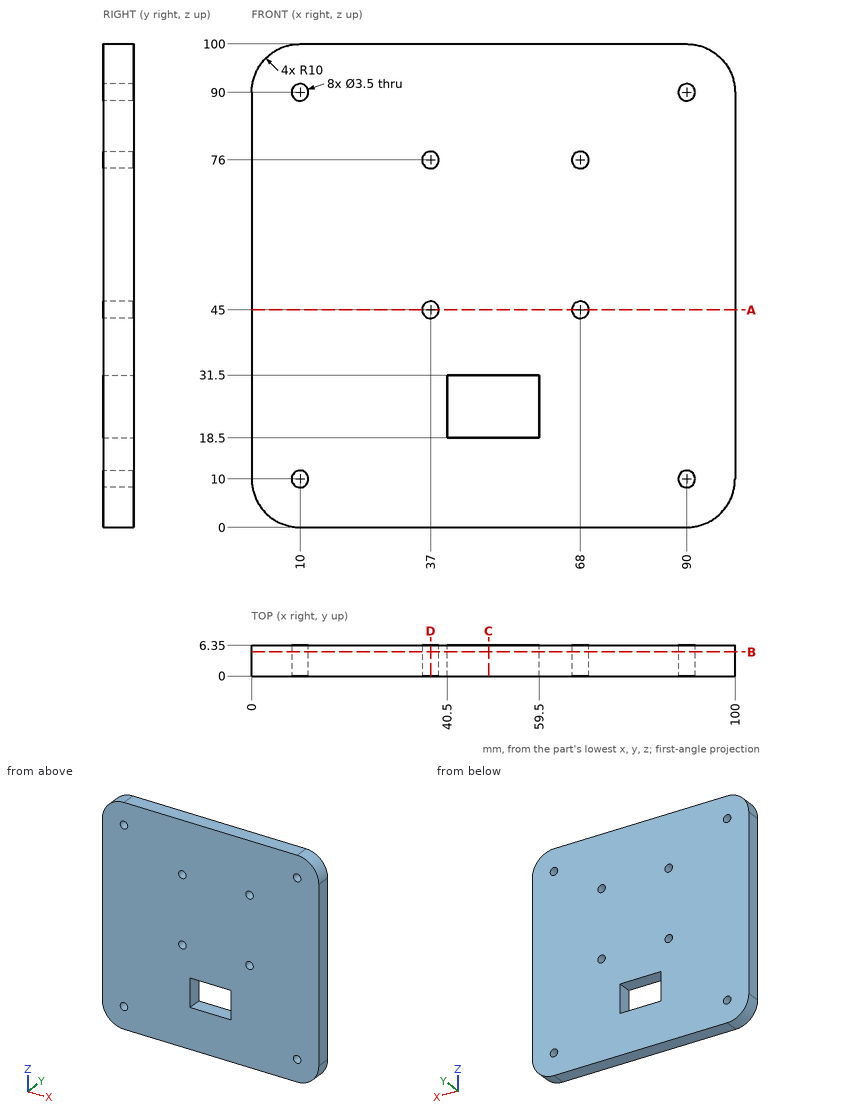
Here's the drawing with two shaded views (mm, measured from the low corner). I have some questions. Coordinates: 2 decimals unless noted, no trailing zeros. Order: outer loops, then holes, each group sorted by start corner. A loop starts at its lowest first (then second) coordinate and runs counter-clockwise, first axis right, second up.
Q1. Suppose I cut it at A-A on z = 45. Please give me the cut outline in (x, y).
Q2. Will these pins go through, and if not, where does the flat tip stop? pin 1 (3 mm diameter, centred on x = 37, z = 45, fed in from -Y); pin 2 (4 mm diameter, centred on x = 68, z = 45, fed in from +Y).
Q3. Please list where these lines run through material, in increasing order: L1, parallel to X at y = 4.25, z = 76; L2, parallel to Z at x = 68, y = 3.75; L3, parallel to X at y = 2.5, z = 27.5.
Q4. Suppose I cut it at C-C on x = 49. Please give me the cut outline in (y, z), and give its area (3 significant figures).
Q5. Suppose I cut it at D-D on x = 37. Please give me the cut outline in (y, z).
Q6. Suppose I cut it at B-B on y = 5. Give the number of separate pieces and of enclosed holes in the cut face, and give its area (3 significant figures).
Answer:
1. outline: (0, 0) - (35.25, 0) - (35.25, 6.35) - (0, 6.35) - close; (38.75, 0) - (66.25, 0) - (66.25, 6.35) - (38.75, 6.35) - close; (69.75, 0) - (100, 0) - (100, 6.35) - (69.75, 6.35) - close
2. pin 1: passes through
2. pin 2: stops at y = 6.35
3. L1: x = 0 to 35.25, 38.75 to 66.25, 69.75 to 100
3. L2: z = 0 to 43.25, 46.75 to 74.25, 77.75 to 100
3. L3: x = 0 to 40.5, 59.5 to 100
4. outline: (0, 0) - (6.35, 0) - (6.35, 18.5) - (0, 18.5) - close; (0, 31.5) - (6.35, 31.5) - (6.35, 100) - (0, 100) - close
4. area: 552 mm2
5. outline: (0, 0) - (6.35, 0) - (6.35, 43.25) - (0, 43.25) - close; (0, 46.75) - (6.35, 46.75) - (6.35, 74.25) - (0, 74.25) - close; (0, 77.75) - (6.35, 77.75) - (6.35, 100) - (0, 100) - close
6. separate pieces: 1
6. enclosed holes: 9
6. area: 9,590 mm2
